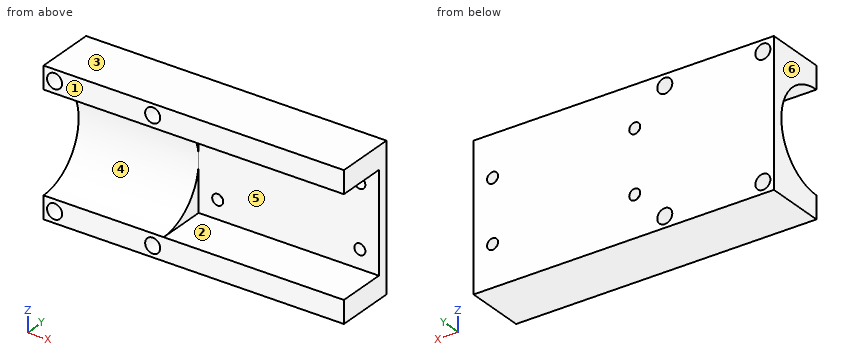
from build123d import *

# Parameters (mm, degrees)
SKETCH1_W           = 30
SKETCH1_H           = 36
BOSS_EXTRUDE1_DEPTH = 30
SKETCH3_R           = 12.375
CUT_EXTRUDE1_DEPTH  = 40
SKETCH5_R           = 1.875
CUT_EXTRUDE2_DEPTH  = 40
CUT_EXTRUDE3_START  = 15
SKETCH7_W           = 36
SKETCH7_H           = 15
CUT_EXTRUDE3_DEPTH  = 31
BOSS_EXTRUDE2_DEPTH = 45
SKETCH9_R           = 1.375
CUT_EXTRUDE4_DEPTH  = 10


with BuildPart() as part:
    # Sketch1 → Boss-Extrude1 (new body)
    with BuildSketch(Plane(origin=(0, 0, 0), x_dir=(1, 0, 0), z_dir=(0, 1, 0))):
        Rectangle(SKETCH1_W, SKETCH1_H)
    extrude(amount=BOSS_EXTRUDE1_DEPTH)

    # Sketch3 → Cut-Extrude1 (cut)
    with BuildSketch(Plane(origin=(15, 0, 0), x_dir=(0, 0, -1), z_dir=(1, 0, 0))):
        with Locations((0, 15)):
            Circle(SKETCH3_R)
    extrude(amount=-CUT_EXTRUDE1_DEPTH, mode=Mode.SUBTRACT)

    # Sketch5 → Cut-Extrude2 (cut)
    with BuildSketch(Plane(origin=(0, 30, 0), x_dir=(1, 0, 0), z_dir=(0, 1, 0))):
        with Locations((-12.25, 15.25)):
            Circle(SKETCH5_R)
        with Locations((-12.25, -15.25)):
            Circle(SKETCH5_R)
        with Locations((12.25, -15.25)):
            Circle(SKETCH5_R)
        with Locations((12.25, 15.25)):
            Circle(SKETCH5_R)
    extrude(amount=-CUT_EXTRUDE2_DEPTH, mode=Mode.SUBTRACT)

    # Sketch7 → Cut-Extrude3 (cut, through all)
    with BuildSketch(Plane(origin=(0, 0, 0), x_dir=(0, 0, -1), z_dir=(1, 0, 0)).offset(CUT_EXTRUDE3_START)):
        with Locations((0, 7.5)):
            Rectangle(SKETCH7_W, SKETCH7_H)
    extrude(amount=-CUT_EXTRUDE3_DEPTH, mode=Mode.SUBTRACT)

    # Sketch8 → Boss-Extrude2 (add)
    with BuildSketch(Plane(origin=(15, 0, 0), x_dir=(0, 0, -1), z_dir=(1, 0, 0))):
        Polygon((-18, 30), (18, 30), (18, 27.331397605), (18, 15), (12.375, 15), (12.375, 27.331397605), (-12.375, 27.331397605), (-12.375, 15), (-18, 15), (-18, 27.331397605), align=None)
    extrude(amount=BOSS_EXTRUDE2_DEPTH)

    # Sketch9 → Cut-Extrude4 (cut)
    with BuildSketch(Plane(origin=(0, 30, 0), x_dir=(1, 0, 0), z_dir=(0, 1, 0))):
        with Locations((19.75, 7.75)):
            Circle(SKETCH9_R)
        with Locations((19.75, -7.75)):
            Circle(SKETCH9_R)
        with Locations((55.25, -7.75)):
            Circle(SKETCH9_R)
        with Locations((55.25, 7.75)):
            Circle(SKETCH9_R)
    extrude(amount=-CUT_EXTRUDE4_DEPTH, mode=Mode.SUBTRACT)


solid = part.part
Geometry: final body of the model. Coordinates: model frame, mm. Face numbers are marked on the shaded views. A direction names the side the tool comes from. Round coordinates to 2 decimals unless told otherwise and drop trailing zeros. Loops run counter-clockwise (first coordinate to the right, second up) from the corner with the lowest first, then second, coordinate; pieces in that order, holes last. Notation, with made-up numbers: M 77.5,6 L 109.5,6 A19 ccw 109.5,28 Z; hole C 28.5,-28 d4. An arc over 180 degrees is marked long. One line per question, with ' | ' between items.
(1) Cut plane B-B on y = 24.25. Return the cut outline in (x, z) (3 decimals).
Check result:
outline: M -15,-18 L 60,-18 L 60,-12.375 L 15,-12.375 L 15,-8.221 L -15,-8.221 Z; M -15,8.221 L 15,8.221 L 15,12.375 L 60,12.375 L 60,18 L -15,18 Z; hole C -12.25,-15.25 d3.75; hole C -12.25,15.25 d3.75; hole C 12.25,-15.25 d3.75; hole C 12.25,15.25 d3.75
(2) Access query for the marked faces 1 and 2. Directions: +Z, -Z, +X, -X, +Y, -Y. A direction counts if a zero-diameter tool reaches every point of the face in a straight line with its end or side. Return the directions, or none.
Check result:
face 1: +Z, -Z, +X, -X, -Y | face 2: +X, -Y
(3) Cut plane A-A on x = 12.25. Return the cut outline in (y, z) (3 decimals), plus the area to 3 significant figures.
Check result:
outline: M 15,-18 L 30,-18 L 30,-17.125 L 15,-17.125 Z; M 15,-13.375 L 30,-13.375 L 30,13.375 L 15,13.375 L 15,12.375 A12.375 cw 15,-12.375 Z; M 15,17.125 L 30,17.125 L 30,18 L 15,18 Z | area: 187 mm2
(4) Material intervals for line 1 along Z through (x, y) = (19.75, 28.85) (3 decimals); line 2 along X through (y, z) = (24.5, -15.25) (3 decimals); line 3 along Z through (x, y) = (43.5, 20.75) (3 decimals), sorted ascending. Write a range as from..to.
Check result:
line 1: z = -18..-9.125, -6.375..6.375, 9.125..18 | line 2: x = -15..-14.125, -10.375..10.375, 14.125..60 | line 3: z = -18..-12.375, 12.375..18
(5) Cut plane D-D on x = 55.25. Return the cut outline in (y, z) (3 decimals).
Check result:
outline: M 15,-18 L 30,-18 L 30,-9.125 L 27.331,-9.125 L 27.331,-12.375 L 15,-12.375 Z; M 15,12.375 L 27.331,12.375 L 27.331,9.125 L 30,9.125 L 30,18 L 15,18 Z; M 27.331,-6.375 L 30,-6.375 L 30,6.375 L 27.331,6.375 Z
(6) Pull-direction query (Z, two-part tool) for the marked faces 3, 4, 5 and 6; classes: +Z half, -Z half, draft (parallel to the pull), parting line (faces both ways), or undercut.
Check result:
face 3: +Z half | face 4: undercut | face 5: undercut | face 6: draft
(7) Contact query for flat-ended pins moving along their axis: P1, Ø6, axis at x = 12.25, z = -15.25, coming from the -Y side; P2, Ø2, axis at x = -12.25, z = 15.25, coming from the +Y side; P3, Ø3.5, axis at x = 55.25, z = -7.75, coming from the -Y side; P4, Ø1.5, axis at x = 15.5, z = -5, coming from the -Y side. Output: stop coordinate, or through.
Check result:
P1: stops at y = 15 | P2: passes through | P3: stops at y = 27.33 | P4: stops at y = 26.06
(8) Cut plane C-C on z = -15.25. Return the cut outline in (x, y) (3 decimals), plus the area to 3 significant figures.
Check result:
outline: M -15,15 L -14.125,15 L -14.125,30 L -15,30 Z; M -10.375,15 L 10.375,15 L 10.375,30 L -10.375,30 Z; M 14.125,15 L 60,15 L 60,30 L 14.125,30 Z | area: 1,010 mm2
